Autodesk Inventor part; units mm, degrees
ref_plane "YZ Plane" through (0, 0, 0) normal (1, 0, 0) x (0, 1, 0)
ref_plane "XZ Plane" through (0, 0, 0) normal (0, 1, 0) x (-1, 0, 0)
ref_plane "XY Plane" through (0, 0, 0) normal (0, 0, 1) x (1, 0, 0)
sketch "Sketch2" plane through (0, 0, 0) normal (0, 0, 1) x (1, 0, 0)
  line L0 (-40, 16) -> (40, 16)
  line L1 (40, 16) -> (40, -16)
  line L2 (40, -16) -> (-40, -16)
  line L3 (-40, -16) -> (-40, 16)
  line L4 (-40, 16) -> (40, -16) construction
  line L5 (40, 16) -> (-40, -16) construction
  point P0 (0, 0)
  dimension "d4" = 32
  dimension "d5" = 80
extrude "Extrusion1" add sketch "Sketch2" along normal blind 26
sketch "Sketch6" plane through (-40, 16, 0) normal (0, 1, 0) x (1, 0, 0)
  line L0 (12, -9.5) -> (0, -9.5) construction
  line L1 (0, 0) -> (0, -26)
  line L2 (68, -9.5) -> (80, -9.5) construction
  line L3 (80, 0) -> (80, -26)
  line L4 (80, 0) -> (0, 0)
  point P0 (40, 0)
  point P1 (74, -9.5)
  dimension "d29" = 56
  dimension "d30" = 9.5
hole "Hole3" at (-28, 16, 9.5) at (28, 16, 9.5) direction (0, -1, 0) diameter 8.2 end through all
sketch "Sketch7" plane through (0, 0, 26) normal (0, 0, 1) x (1, 0, 0)
  point P0 (0, 0)
  point P1 (0, 0)
hole "Hole4" at (0, 0, 26) direction (0, 0, -1) diameter 14.2 end through all counterbore diameter 16.2 counterbore depth 5.2
sketch "Sketch8" plane through (0, 0, 0) normal (0, 0, -1) x (-1, 0, 0)
  point P0 (0, 0)
  point P1 (0, 0)
hole "Hole5" at (0, 0, 0) direction (0, 0, 1) diameter 14.2 end through all counterbore diameter 16.2 counterbore depth 5.2
sketch "Sketch9" plane through (-40, 16, 0) normal (0, 1, 0) x (1, 0, 0)
  line L0 (0, 0) -> (0, -26)
  line L1 (80, -26) -> (0, -26)
  line L2 (0, 0) -> (80, -26)
  point P0 (40, 0)
sketch "Sketch10" plane through (-40, 16, 0) normal (0, 1, 0) x (1, 0, 0)
  point P0 (40, 0)
sketch "Sketch11" plane through (40, -16, 0) normal (1, 0, 0) x (0, 0, -1)
  line L0 (0, 0) -> (0, 32)
  line L1 (0, 0) -> (-26, 0)
  line L2 (-26, 0) -> (-26, 200)
  line L3 (-26, 200) -> (0, 200)
  line L4 (0, 200) -> (0, 0)
  line L5 (-26, 0) -> (-26, 32)
  point P0 (0, 16)
  dimension "d52" = 200
extrude "Extrusion4" add sketch "Sketch11" along normal blind 32
fillet "Fillet1" radius 10 1 edges at (72, -16, 13)
sketch "Sketch13" plane through (40, 184, 26) normal (0, 1, 0) x (1, 0, 0)
  line L0 (32, 26) -> (-30, 26)
  line L1 (0, 26) -> (-80, 26)
  line L2 (32, 26) -> (32, 0)
  line L3 (32, 26) -> (32, -36)
  line L4 (-30, 26) -> (32, -36)
  point P0 (-40, 26)
  dimension "d58" = 62
extrude "Extrusion5" add sketch "Sketch13" against normal blind 10
fillet "Fillet2" radius 5 1 edges at (10, 179, 0)
fillet "Fillet3" radius 5 1 edges at (72, 179, 62)
sketch "Sketch15" plane through (22.0711, 184, 0) normal (0, 1, 0) x (1, 0, 0)
  line L0 (0, 0) -> (49.9289, 0)
  line L1 (49.9289, 0) -> (49.9289, -26)
  line L2 (49.9289, 0) -> (17.9289, 0)
  line L3 (17.9289, 0) -> (17.9289, -32)
  line L4 (17.9289, -32) -> (49.9289, -32)
  line L5 (49.9289, -32) -> (49.9289, 0)
  line L6 (49.9289, 0) -> (49.9289, -49.9289)
  point P0 (-22.0711, 0)
  point P1 (41.9289, -42)
  point P2 (7.9289, -8)
  dimension "d63" = 8
  dimension "d64" = 32
  dimension "d65" = 32
  dimension "d66" = 10
  dimension "d67" = 10
  dimension "d68" = 8
hole "Hole6" at (30, 184, 8) at (64, 184, 42) direction (0, -1, 0) diameter 8.2 depth 20
properties part number "13042026-07"
Geometry: final body of the model. Coordinates: model frame, mm. A direction names the side the tool comes from. Give positions to 0.01 mm unless a question says otherwise; leave off trailing zeros. Write each loop counter-clockwise with the first axis right and the second up, starting at its lowest first coordinate (ties: lowest second). Pieces come first, ordered by that corner, then holes. Notation, with made-up numbers: (36, 32.25) - (55, 32.25) arc R16 cw to (55, 37.25) - close; hole circle Ø10 at (49, -0.75). An arc over 180 degrees is marked (long way). Return JSON: item names as keys, results as strings. Group by question number.
1) First-contact query: P1, Ø18, axis at x = 1, y = -2.5, coming from the +Z side; P2, Ø5, axis at x = 30, z = 8, coming from the +Y side; P3, Ø14.5, axis at x = 0, y = 0, coming from the -Z side. Flat tips, straight axial feed; report the tip coordinate or a pass-through.
2) Section B-B on x = 28. Return the cut outline in (y, z), plus the area to 3 significant figures.
3) Section A-A on x = -28. Return the cut outline in (y, z), plus the area to 3 significant figures.
4) Section C-C on y = 73. Return the cut outline in (x, z).
5) Section D-D on z = 48. Return the cut outline in (x, y), plus the area to 3 significant figures.
6) Mould query, pull axis Y, two halves, no side actions, for faces 4 (the cylindrical face through (7.907, -1.756, 2.636)), 5 (the cylindrical face through (68.99, -13.15, 13.18)), 6 (the flat face through (-40, 0, 13)), 7 (the flat face through (-1, 16, 13)). Classes: released by +Y, released by -Y, zero draft, split by the parting line, or undercut.
7) Set-up query: faces 1 (the cylindrical face through (34, 178.9, 7.1)), 2 (the flat face through (41, 179, 31)), 3 (the cylindrical face through (17.42, 178.93, 3.16)). Return all of +Z, -Z, +X, -X, +Y, -Y with unobstructed straight access to the full face (end or side cutting, diameter ignored); none if empty.
8) Line query: line 1 (Y direction, x = 34, z = 3); line 2 (X direction, y = -3, z = 9.5); line 3 (Y direction, x = 0, z = 22). Output: solid intervals per line, ascending.
Filled in:
{
 "1": {"P1": "stops at z = 26", "P2": "stops at y = 16", "P3": "stops at z = 5.2"},
 "2": {"outline": "(-16, 0) - (16, 0) - (16, 5.4) - (-16, 5.4) - close; (-16, 13.6) - (16, 13.6) - (16, 26) - (-16, 26) - close; (174, 0) - (184, 0) - (184, 4.42) - (174, 4.42) - close; (174, 11.58) - (184, 11.58) - (184, 18) - (174, 18) - close", "area": "678 mm^2"},
 "3": {"outline": "(-16, 0) - (16, 0) - (16, 5.4) - (-16, 5.4) - close; (-16, 13.6) - (16, 13.6) - (16, 26) - (-16, 26) - close", "area": "570 mm^2"},
 "4": {"outline": "(40, 0) - (72, 0) - (72, 26) - (40, 26) - close"},
 "5": {"outline": "(58, 174) - (72, 174) - (72, 184) - (58, 184) - close", "area": "140 mm^2"},
 "6": {"face 4": "undercut", "face 5": "released by -Y", "face 6": "zero draft", "face 7": "undercut"},
 "7": {"face 1": "+Y", "face 2": "+Z, -X, +Y", "face 3": "-X, +Y"},
 "8": {"line 1": "y = -16 to 16, 174 to 184", "line 2": "x = -40 to -32.1, -23.9 to -6.44, 6.44 to 23.9, 32.1 to 72", "line 3": "y = -16 to -8.1, 8.1 to 16"}
}
